Geometry check sheet. Reference: drawing and pictorial views, mm from the part's lowest x, y, z. Coordinates: 2 decimals unless noted, no trailing zeros. Loops run counter-clockwise (first coordinate to the right, second up) from the corner with the lowest first, then second, coordinate; pieces in that order, holes last. Notation, with made-up numbers: (-33.5, -23) -> (-29.5, -23) arc R28 ccw to (-29.5, 7) -> close; hole circle Ø7 at (17, -18). An arc over 180 degrees is marked (long way). Answer as a JSON object with one key per item and string values. Group by question number.
Q1. Cross-section at B-B on y = 220. Record the boundary of the cut face in (x, z).
Q2. Scan lines: L1, parallel to X at y = 621.5, z = 21.25; L2, parallel to X at y = 271.5, z = 13.25; L3, parallel to Y at x = 568.5, z = 8. Record each from-to range of solid material in increasing order.
Q3. Cross-section at C-C on x = 675.5. Record the boundary of the cut face in (y, z), and give its area (3 significant figures).
Q4. Gauge pin test, flat end, axial feed: pin 1 Ø5 at (y, z) = (267.5, 17.5) entering from -X. Record the tip position at first contact, or that the pin passes through.
Q5. Cross-section at A-A on z = 20.25. Record the boundary of the cut face in (x, y), and give its area (3 significant figures).
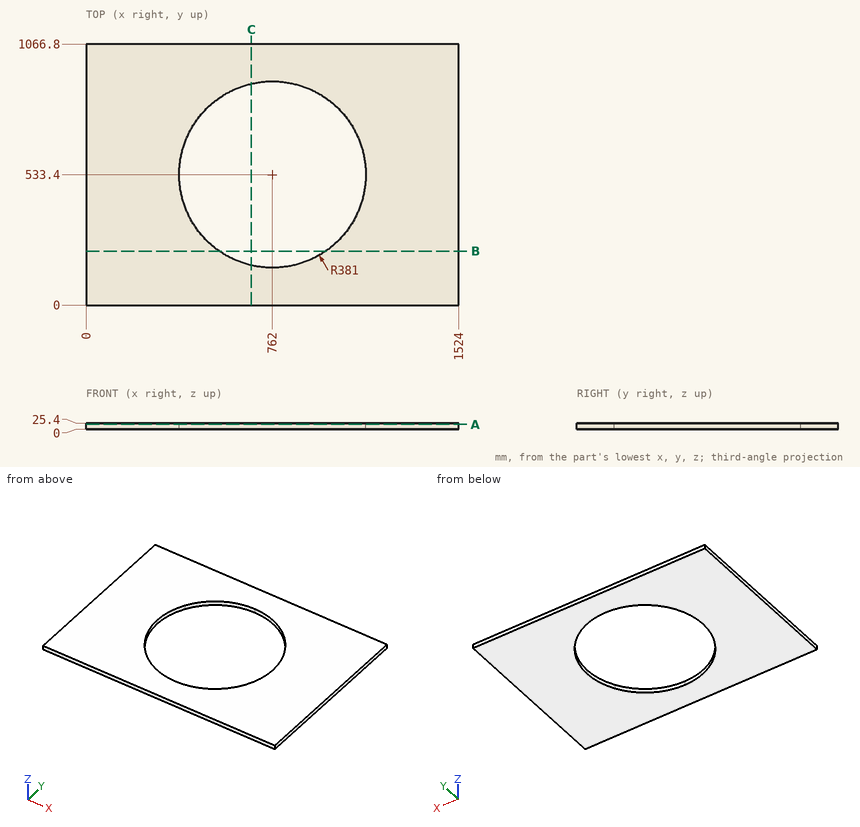
Computed values:
{
 "1": {"outline": "(0, 0) -> (545.34, 0) -> (545.34, 25.4) -> (0, 25.4) -> close; (978.66, 0) -> (1524, 0) -> (1524, 25.4) -> (978.66, 25.4) -> close"},
 "2": {"L1": "x = 0 to 391.33, 1132.67 to 1524", "L2": "x = 0 to 485.29, 1038.71 to 1524", "L3": "y = 0 to 205.19, 861.61 to 1066.8"},
 "3": {"outline": "(0, 0) -> (162.35, 0) -> (162.35, 25.4) -> (0, 25.4) -> close; (904.45, 0) -> (1066.8, 0) -> (1066.8, 25.4) -> (904.45, 25.4) -> close", "area": "8,250 mm²"},
 "4": {"pin 1": "stops at x = 0"},
 "5": {"outline": "(0, 0) -> (1524, 0) -> (1524, 1066.8) -> (0, 1066.8) -> close; hole (381, 533.4) arc R381 ccw to (431.8, 343.32) arc R381 ccw to (1092.2, 343.32) arc R381 ccw to (1143, 533.4) arc R381 ccw to (1092.2, 723.48) arc R381 ccw to (431.8, 723.48) arc R381 ccw to start", "area": "1,170,000 mm²"}
}
